from build123d import *

# Parameters (mm, degrees)
SKETCH1_R                = 1.05
BOSS_EXTRUDE1_DEPTH      = 3
BOSS_EXTRUDE2_DEPTH      = 4
BOSS_EXTRUDE2_DEPTH_BACK = 4
LOFT2_START              = -4
LOFT2_DEPTH              = 8
FILLET1_R                = 3
CUT_EXTRUDE1_DEPTH       = 49.748957751
CUT_EXTRUDE1_DEPTH_BACK  = 49.748957751
SKETCH8_R                = 1.05
CUT_EXTRUDE2_DEPTH       = 0.8


# Read off the part's stored shape, not the designer's step: Loft2
with BuildPart() as part:
    # Sketch1 → Boss-Extrude1 (new body)
    with BuildSketch(Plane(origin=(0, 0, 0), x_dir=(1, 0, 0), z_dir=(0, 1, 0))):
        with BuildLine():
            Line((-6.715, -4), (6.715, -4))
            ThreePointArc((6.715, -4), (8.129213562, -3.414213562), (8.715, -2))
            Line((8.715, -2), (8.715, 2))
            ThreePointArc((8.715, 2), (8.129213562, 3.414213562), (6.715, 4))
            Line((6.715, 4), (-6.715, 4))
            Line((-6.715, 4), (-11.585, 4))
            Line((-11.585, 4), (-11.585, -4))
            Line((-11.585, -4), (-6.715, -4))
        make_face()
        with Locations(Location((-5.715, 0, 0), (0, 0, 270))):
            Circle(SKETCH1_R, mode=Mode.SUBTRACT)
        with Locations(Location((5.715, 0, 0), (0, 0, 270))):
            Circle(SKETCH1_R, mode=Mode.SUBTRACT)
    extrude(amount=BOSS_EXTRUDE1_DEPTH)



with BuildPart() as body_2:
    # Sketch3 → Boss-Extrude2 (new, two sides: drawn at the far end of the back side and taken through both)
    with BuildSketch(Plane.XY.offset(-BOSS_EXTRUDE2_DEPTH_BACK)):
        with BuildLine():
            Line((-41.354696007, 22.5), (-41.354696007, 21.5))
            Line((-41.354696007, 21.5), (-41.354696007, 20.5))
            Line((-41.354696007, 20.5), (-36.354696007, 20.5))
            Line((-36.354696007, 20.5), (-35.915127019, 20.5))
            ThreePointArc((-35.915127019, 20.5), (-34.085, 18.669872981), (-31.585, 18))
            Line((-31.585, 18), (-26.585, 18))
            Line((-26.585, 18), (-26.585, 23))
            ThreePointArc((-26.585, 23), (-30.290904774, 27.829629131), (-35.915127019, 25.5))
            Line((-35.915127019, 25.5), (-36.354696007, 25.5))
            Line((-36.354696007, 25.5), (-41.354696007, 25.5))
            Line((-41.354696007, 25.5), (-41.354696007, 24.5))
            Line((-41.354696007, 24.5), (-41.354696007, 23.5))
            Line((-41.354696007, 23.5), (-36.354696007, 23.5))
            Line((-36.354696007, 23.5), (-35.049101615, 23.5))
            ThreePointArc((-35.049101615, 23.5), (-31.334356481, 26.491013868), (-28.085, 23))
            ThreePointArc((-28.085, 23), (-31.334356481, 19.508986132), (-35.049101615, 22.5))
            Line((-35.049101615, 22.5), (-36.354696007, 22.5))
            Line((-36.354696007, 22.5), (-41.354696007, 22.5))
        make_face()
    extrude(amount=BOSS_EXTRUDE2_DEPTH + BOSS_EXTRUDE2_DEPTH_BACK)


with BuildPart() as part_1:
    add(part.part)

    add(body_2.part)  # Loft2 merges body 2
    # Loft2 outline → Loft2 (add)
    with BuildSketch(Plane.XY.offset(LOFT2_START)):
        Polygon((-11.585, 3), (-26.585, 18), (-31.585, 18), (-11.585, 0), align=None)
    extrude(amount=LOFT2_DEPTH)

    # Fillet1
    fillet1_edges = [part_1.edges().sort_by_distance(p)[0] for p in [
        (-31.585, 18, 0),
        (-26.585, 18, 0),
        (-11.585, 3, 0),
    ]]
    fillet(fillet1_edges, radius=FILLET1_R)

    # Sketch8 → Cut-Extrude1 (cut, two sides: drawn at the far end of the back side and taken through both)
    with BuildSketch(Plane(origin=(0, 25.5, 0), x_dir=(1, 0, 0), z_dir=(0, 1, 0)).offset(-CUT_EXTRUDE1_DEPTH_BACK)):
        with Locations(Location((-38.59424289, 0, 0), (0, 0, 90))):
            Circle(SKETCH8_R)
    extrude(amount=CUT_EXTRUDE1_DEPTH + CUT_EXTRUDE1_DEPTH_BACK, mode=Mode.SUBTRACT)

    # Sketch9 → Cut-Extrude2 (cut)
    with BuildSketch(Plane.XZ.offset(-20.5)):
        Polygon((-36.59424289, 1.154700538), (-38.59424289, 2.309401077), (-40.59424289, 1.154700538), (-40.59424289, -1.154700538), (-38.59424289, -2.309401077), (-36.59424289, -1.154700538), align=None)
    extrude(amount=-CUT_EXTRUDE2_DEPTH, mode=Mode.SUBTRACT)


solid = part_1.part
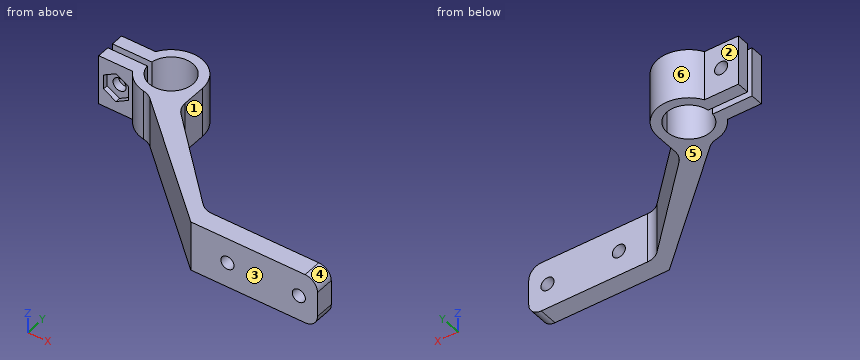
CAD build for the part. Positions are in the model's coordinates, mm. Face numbers are marked on the shaded views. A direction names the side the tool comes from. Round coordinates to 2 decimals unless told otherwise and drop trailing zeros. Write each loop counter-clockwise with the first axis right and the second up, starting at its lowest first coordinate (ties: lowest second). Pieces come first, ordered by that corner, then holes.
(1) Drop flat-ended pins along their axis: P1, Ø4.5, axis at x = -37.5, z = 0, coming from the -Y side; P2, Ø1.5, axis at x = -33, z = -1, coming from the -Y side; P3, Ø4, axis at y = 9, z = -3, coming from the -X side. Give the stop position or say it passes through.
(2) Probe line 1 along X through (y, z) = (24.35, 0); line 2 along X through (y, z) = (24, 0); line 3 along Y through (x, z) = (4, 0.75). List the from-to ranges inside material, lowest first.
(3) Slice it at D-D, the plane z = -3. Write the cut outline in (x, y) (3 decimals).
(4) Slice it at B-B, the plane z = 0. Count the separate pieces of the cut face and the enclosed holes in it, and give its area (3 significant figures).
(5) Mould opens along Z. For the marked faces 4, 5 and 6 say: pulls with the +Z half, pulls with the -Z half, needs draft (parallel to the pull), parting line crosses it, or undercut.
(6) Slice it at A-A, the plane y = 24.25. Write the cut outline in (x, z), and give its area (3 significant figures).
(7) 3-axis set-ups, long thin cutter, end or side, ignore diameter. For the marked faces 1, 2 and 3: which of +Z, -Z, +X, -X, +Y, -Y reach the whole face in a straight line?
(8) Slice it at C-C, the plane x = 2. Write the cut outline in (y, z), and give its area (3 significant figures).
From the geometry:
1. P1: stops at y = 19.6
1. P2: stops at y = 18.04
1. P3: stops at x = -23.81
2. line 1: x = -41.35 to -39.64, -37.54 to -34.81, -28.36 to -26.77
2. line 2: x = -41.35 to -39.64, -37.54 to -34.94, -28.23 to -26.69
2. line 3: y = 0 to 3
3. outline: (-41.355, 20.5) - (-35.915, 20.5) arc R5 ccw to (-32.374, 18.063) arc R3 cw to (-30.841, 17.33) - (-11.585, 0) - (8.447, 0) - (8.447, 3) - (-10.342, 3) arc R3 cw to (-12.464, 3.879) - (-25.706, 17.121) arc R3 cw to (-26.585, 19.243) - (-26.585, 23) arc R5 ccw to (-35.915, 25.5) - (-41.355, 25.5) - (-41.355, 23.5) - (-35.049, 23.5) arc R3.5 cw (long way) to (-35.049, 22.5) - (-41.355, 22.5) - close
4. separate pieces: 5
4. enclosed holes: 0
4. area: 170 mm2
5. face 4: pulls with the +Z half
5. face 5: pulls with the -Z half
5. face 6: needs draft
6. outline: (-41.35, -4) - (-34.85, -4) - (-34.85, 4) - (-41.35, 4) - close; (-28.32, -4) - (-26.74, -4) - (-26.74, 4) - (-28.32, 4) - close; hole circle Ø2.1 at (-38.59, 0)
6. area: 61.1 mm2
7. face 1: +Z, -Z, +X, +Y
7. face 2: +Z, -Z, -X, +Y
7. face 3: +Z, -Z, +X, -X, -Y
8. outline: (0, -4) - (3, -4) - (3, 4) - (0, 4) - close
8. area: 24.0 mm2
